Geometry: see drawing. Coordinates: mm, zero at the bounding-box minimum. Coordinates: 2 decimals unless noted, no trailing zeros. Loops run counter-clockwise (first coordinate to the right, second up) from the corner with the lowest first, then second, coordinate; pieces in that order, holes last. Notation, with made-up numbers: (-35.75, 69.5) -> (-23.75, 69.5) arc R27 ccw to (-23.75, 104.5) -> close; hole circle Ø1 at (-40, -23.75). An arc over 180 degrees is marked (long way). Answer as a JSON object with one key per item and string values.
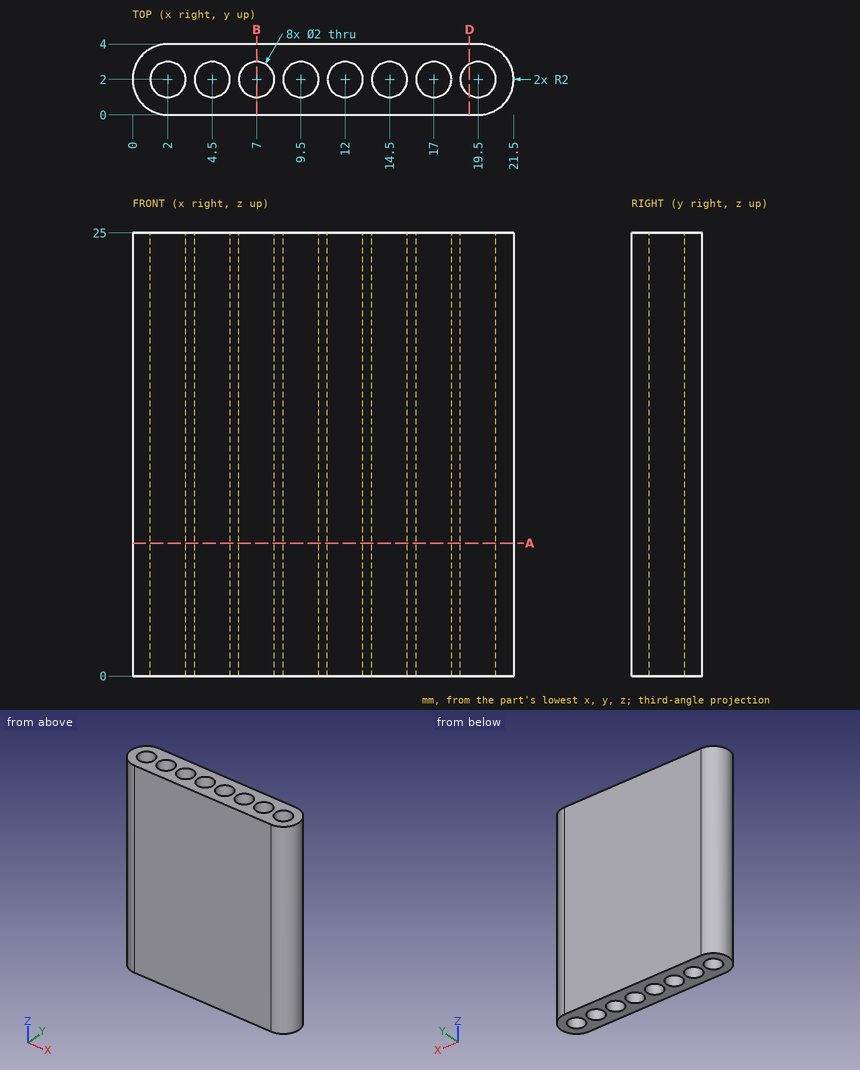
1. Line query: line 1 along Y through (x, z) = (9.5, 19); line 2 along Y through (x, z) = (16.25, 11.25); line 3 along X through (y, z) = (3.5, 20.75). Output: solid intervals per line, ascending.
Reply:
{"line 1": "y = 0 to 1, 3 to 4", "line 2": "y = 0 to 1.34, 2.66 to 4", "line 3": "x = 0.68 to 20.82"}
2. Pin query (flat end, axial travel): P1, Ø1.8, axis at x = 7, y = 2, coming from the +Z side. Return the tip coordinate at first contact, or that it passes through.
Reply:
{"P1": "passes through"}
3. Section query A-A (z = 7.5). Count the separate pieces of the cut face and the enclosed holes in it, plus the area to 3 significant figures.
Reply:
{"separate pieces": "1", "enclosed holes": "8", "area": "57.4 mm2"}
4. Section query B-B (x = 7). Return loops of the section in (y, z), plus the area to 3 significant figures.
Reply:
{"outline": "(0, 0) -> (1, 0) -> (1, 25) -> (0, 25) -> close; (3, 0) -> (4, 0) -> (4, 25) -> (3, 25) -> close", "area": "50.0 mm2"}
5. Section query D-D (x = 19). Return loops of the section in (y, z), plus the area to 3 significant figures.
Reply:
{"outline": "(0, 0) -> (1.13, 0) -> (1.13, 25) -> (0, 25) -> close; (2.87, 0) -> (4, 0) -> (4, 25) -> (2.87, 25) -> close", "area": "56.7 mm2"}
